The listing builds one solid part. Answer for the finished solid, in the listing's coordinates (mm). A direction names the side the tool comes from. Round coordinates to 2 decimals unless told otherwise and drop trailing zeros. Loops run counter-clockwise (first coordinate to the right, second up) from the corner with the lowest first, then second, coordinate; pieces in that order, holes last. Notation, with made-up numbers: M 42.25,28 L 75.25,28 A8 ccw 75.25,37 Z; hole C 43,35.25 d3. An arc over 180 degrees is marked long. Answer as a JSON object with one key per item and string values.
```python
from build123d import *

# Parameters (mm, degrees)
SKETCH_1_R          = 37.5
EXTRUDE_1_DEPTH     = 12
SKETCH_2_R          = 24.25
EXTRUDE_2_DEPTH     = 105
CHAMFER_1_SIZE      = 35
CHAMFER_1_SIZE2     = 4.607837416
CUT_EXTRUDE_3_DEPTH = 178.024009671
SKETCH_6_R          = 10
EXTRUDE_4_DEPTH     = 12
SKETCH_7_R          = 5
CUT_EXTRUDE_5_DEPTH = 122.191996522


with BuildPart() as part:
    # 草图1 → 拉伸1 (new body)
    with BuildSketch(Plane.XY):
        Circle(SKETCH_1_R)
    extrude(amount=EXTRUDE_1_DEPTH)

    # 草图2 → 拉伸2 (add)
    with BuildSketch(Plane(origin=(0, 0, 0), x_dir=(-1, 0, 0), z_dir=(0, 0, -1))):
        with Locations(Location((0, 0, 0), (0, 0, 180))):
            Circle(SKETCH_2_R)
    extrude(amount=EXTRUDE_2_DEPTH)

    # 倒角1
    chamfer_1_edges = [part.edges().sort_by_distance(p)[0] for p in [
        (-24.25, 0, -105),
    ]]
    chamfer_1_side = [part.faces().sort_by_distance(p)[0] for p in [
        (-24.25, 0, -52.5),
    ]]
    chamfer(chamfer_1_edges, length=CHAMFER_1_SIZE, length2=CHAMFER_1_SIZE2, reference=chamfer_1_side[0])

    # 草图3 → 拉伸3 (cut, through all)
    with BuildSketch(Plane(origin=(100, 0, 0), x_dir=(0, 0, -1), z_dir=(1, 0, 0))):
        with BuildLine():
            Line((60, 5), (70, 5))
            ThreePointArc((70, 5), (75, 0), (70, -5))
            Line((70, -5), (60, -5))
            Line((60, -5), (60, 5))
        make_face()
    extrude(amount=-CUT_EXTRUDE_3_DEPTH, mode=Mode.SUBTRACT)

    # 草图6 → 拉伸4 (add)
    with BuildSketch(Plane(origin=(0, 0, 0), x_dir=(-1, 0, 0), z_dir=(0, 0, -1))):
        with Locations((0, 37.5)):
            Circle(SKETCH_6_R)
    extrude(amount=-EXTRUDE_4_DEPTH)

    # 草图7 → 拉伸5 (cut, through all)
    with BuildSketch(Plane(origin=(0, 0, 0), x_dir=(-1, 0, 0), z_dir=(0, 0, -1))):
        with Locations((0, 37.5)):
            Circle(SKETCH_7_R)
    extrude(amount=-CUT_EXTRUDE_5_DEPTH, mode=Mode.SUBTRACT)


solid = part.part
```
Item 1: Flat-ended cylindrical pins translate along their axes: P1, Ø1.5, axis at x = -9, z = -37, coming from the +Y side; P2, Ø5, axis at y = 1.5, z = -64, coming from the -X side; P3, Ø8, axis at y = 22.5, z = -52.5, coming from the -X side; P4, Ø13, axis at x = 0, y = 37.5, coming from the -Z side. Find the tip coordinate at first contact, or state that the pin passes through.
Values follow:
{"P1": "y = 22.8", "P2": "through", "P3": "x = -15.68", "P4": "z = 0"}
Item 2: The part is cut by section C-C (z = -2.5). Give the vertices of the cut face in (x, y).
Values follow:
{"outline": "C 0,0 d48.5"}
Item 3: Determine the mould class of faces 1 (the face through (20.414, -6.429, -91.634)), 2 (the face through (0, 5, -65)), 3 (the face through (0.651, 42.457, 5.916)) for opening direction Z: released by +Z, released by -Z, zero draft, split by the parting line, or undercut.
Values follow:
{"face 1": "released by -Z", "face 2": "undercut", "face 3": "zero draft"}
Item 4: Which of the six approach directions +Z, -Z, +X, -X, +Y, -Y give full straight-line access (tool end or side, diameter ignored) to faces 4 (the face through (1, -4, 12)), 5 (the face through (0.5, 24.5, 0)), 6 (the face through (0, 0, -60))?
Values follow:
{"face 4": "+Z, +X, -X, +Y, -Y", "face 5": "-Z", "face 6": "+X, -X"}
Item 5: The part is cut by section A-A (x = 0). Give the vertices of the cut face in (y, z).
Values follow:
{"outline": "M -37.5,0 L -24.25,0 L -24.25,-70 L -19.64,-105 L 19.64,-105 L 24.25,-70 L 24.25,0 L 32.5,0 L 32.5,12 L -37.5,12 Z; M 42.5,0 L 47.5,0 L 47.5,12 L 42.5,12 Z; hole M -5,-70 A5 ccw 5,-70 L 5,-60 L -5,-60 Z"}
Item 6: Straight lines are drawn through the part: line 1 (Y direction, x = 0, z = 3); line 2 (X direction, y = 38, z = 6.5); line 3 (Z direction, x = 6.5, y = 37). For each, find the intervals that lie inside material, in ascending order.
Values follow:
{"line 1": "-37.5 to 32.5, 42.5 to 47.5", "line 2": "-9.99 to -4.97, 4.97 to 9.99", "line 3": "0 to 12"}
Item 7: The part is cut by section B-B (y = 37.5). Give the vertices of the cut face in (x, z), then the cut area to 3 significant figures.
Values follow:
{"outline": "M -10,0 L -5,0 L -5,12 L -10,12 Z; M 5,0 L 10,0 L 10,12 L 5,12 Z", "area": "120 mm^2"}
Item 8: The part is cut by section D-D (y = 0). Give the vertices of the cut face in (x, z).
Values follow:
{"outline": "M -37.5,0 L -24.25,0 L -24.25,-60 L 24.25,-60 L 24.25,0 L 37.5,0 L 37.5,12 L -37.5,12 Z; M -23.59,-75 L -19.64,-105 L 19.64,-105 L 23.59,-75 Z"}
